The listing builds one solid part. Answer for the finished solid, in the listing's coordinates (mm). A direction names the side the tool comes from. Give positions to 0.01 mm unless a question says otherwise; leave off trailing zeros. Write each loop counter-clockwise with the first axis right and the second up, starting at its lowest first coordinate (ties: lowest second). Pieces come first, ordered by that corner, then holes. Notation, with made-up numbers: M 84,-13.5 L 107,-13.5 A14 ccw 107,-5.5 Z; hole C 15,61 d9. An arc over 180 degrees is marked long. Answer as a JSON object with one key per item and string values.
```python
from build123d import *

# Parameters (mm, degrees)
SKETCH_2_W          = 150
SKETCH_2_H          = 100
EXTRUDE_1_DEPTH     = 90
SKETCH_3_W          = 150
SKETCH_3_H          = 70
CUT_EXTRUDE_1_DEPTH = 80
EXTRUDE_2_DEPTH     = 100
EXTRUDE_3_DEPTH     = 100
SKETCH_7_W          = 310
SKETCH_7_H          = 140
EXTRUDE_4_DEPTH     = 5


with BuildPart() as part:
    # 草图2 → 凸台-拉伸1 (new body)
    with BuildSketch(Plane(origin=(0, 0, 0), x_dir=(1, 0, 0), z_dir=(0, 1, 0))):
        Rectangle(SKETCH_2_W, SKETCH_2_H)
    extrude(amount=EXTRUDE_1_DEPTH)

    # 草图3 → 切除-拉伸1 (cut)
    with BuildSketch(Plane.XY.offset(50)):
        with Locations((0, 45)):
            Rectangle(SKETCH_3_W, SKETCH_3_H)
    extrude(amount=-CUT_EXTRUDE_1_DEPTH, mode=Mode.SUBTRACT)

    # 草图5 → 凸台-拉伸2 (add)
    with BuildSketch(Plane(origin=(0, 0, -50), x_dir=(-1, 0, 0), z_dir=(0, 0, -1))):
        Polygon((-75, 90), (-135, 0), (-75, 0), align=None)
    extrude(amount=-EXTRUDE_2_DEPTH)

    # 草图6 → 凸台-拉伸3 (add)
    with BuildSketch(Plane(origin=(0, 0, -50), x_dir=(-1, 0, 0), z_dir=(0, 0, -1))):
        Polygon((75, 90), (135, 0), (75, 0), align=None)
    extrude(amount=-EXTRUDE_3_DEPTH)

    # 草图7 → 凸台-拉伸4 (add)
    with BuildSketch(Plane.XZ):
        Rectangle(SKETCH_7_W, SKETCH_7_H)
    extrude(amount=-EXTRUDE_4_DEPTH)


solid = part.part
```
1. Consider line 1 along Y through (x, z) = (72, 34); line 2 along Z through (x, y) = (90, 24); line 3 along Z through (x, y) = (49.5, 78.5). Determine where each line is inside the solid, lowest interval first.
Verdict:
{"line 1": "y = 0 to 10, 80 to 90", "line 2": "z = -50 to 50", "line 3": "z = -50 to -30"}
2. A cutting plane is placed at C-C, the plane z = -9. Give the vertices of the cut face in (x, y).
Verdict:
{"outline": "M -155,0 L 155,0 L 155,5 L 131.67,5 L 75,90 L -75,90 L -131.67,5 L -155,5 Z; hole M -75,10 L 75,10 L 75,80 L -75,80 Z"}
3. Flat-ended cylindrical pins translate along their axes: pin 1 (1.5 mm diameter, centred on y = 18, z = -49.5, fed in from -X); pin 2 (5 mm diameter, centred on x = 110.5, y = 31, fed in from +Z); pin 3 (21 mm diameter, centred on y = 46, z = 10, fed in from -X). Find the tip coordinate at first contact, or state that the pin passes through.
Verdict:
{"pin 1": "stops at x = -123.5", "pin 2": "stops at z = 50", "pin 3": "stops at x = -111.33"}
4. A cutting plane is placed at A-A, the plane y = 54. Give the vertices of the cut face in (x, z), plus the area to 3 significant figures.
Verdict:
{"outline": "M -99,-50 L 99,-50 L 99,50 L 75,50 L 75,-30 L -75,-30 L -75,50 L -99,50 Z", "area": "7,800 mm2"}
5. A cutting plane is placed at D-D, the plane x = 69.5. Give the vertices of the cut face in (y, z), plus the area to 3 significant figures.
Verdict:
{"outline": "M 0,-70 L 5,-70 L 5,-50 L 90,-50 L 90,50 L 80,50 L 80,-30 L 10,-30 L 10,50 L 5,50 L 5,70 L 0,70 Z", "area": "3,600 mm2"}
6. For faces 1 (the flat face through (-1, 45, -30)), 2 (the flat face through (-2, 5, -61)), 3 (the flat face through (-2, 48, -50)), determine the directions among +Z, -Z, +X, -X, +Y, -Y from which every point of the face is accessible in a straight line to the end or side of a thin tool.
Verdict:
{"face 1": "+Z", "face 2": "+Y", "face 3": "-Z, +X, -X, +Y"}
7. The mould has two halves that part along X. Classify faces 4 (the flat face through (19, 7, 50)), 5 (the flat face through (-1, 80, 11)), 6 (the flat face through (103, 48, -1)): released by +X, released by -X, zero draft, split by the parting line, or undercut.
Verdict:
{"face 4": "zero draft", "face 5": "undercut", "face 6": "released by +X"}
8. A cutting plane is placed at B-B, the plane x = -126.5. Give the vertices of the cut face in (y, z), plus the area to 4 significant figures.
Verdict:
{"outline": "M 0,-70 L 5,-70 L 5,-50 L 12.75,-50 L 12.75,50 L 5,50 L 5,70 L 0,70 Z", "area": "1,475 mm2"}
